```python
from build123d import *

# Parameters (mm, degrees)
SKETCH1_W                   = 31.75
SKETCH1_H                   = 8.89
SKETCH1_R                   = 2
BOSS_EXTRUDE1_DEPTH         = 2.54
SKETCH3_W                   = 2.54
SKETCH3_H                   = 8.89
BOSS_EXTRUDE2_DEPTH         = 27
SKETCH4_W                   = 17.08
SKETCH4_H                   = 2.54
CUT_EXTRUDE1_DEPTH          = 2.54
TAP_DRILL_FOR_M4X0_7_TAP1_D = 3.3


with BuildPart() as part:
    # Sketch1 → Boss-Extrude1 (new body)
    with BuildSketch(Plane.XY):
        with Locations((17.5, 25)):
            Rectangle(SKETCH1_W, SKETCH1_H)
        with Locations((17.5, 25)):
            Circle(SKETCH1_R, mode=Mode.SUBTRACT)
    extrude(amount=BOSS_EXTRUDE1_DEPTH)

    # Sketch3 → Boss-Extrude2 (add)
    with BuildSketch(Plane.XY.offset(2.54)):
        with Locations((10.23, 25)):
            Rectangle(SKETCH3_W, SKETCH3_H)
        with Locations((24.77, 25)):
            Rectangle(SKETCH3_W, SKETCH3_H)
    extrude(amount=BOSS_EXTRUDE2_DEPTH)

    # Sketch4 → Cut-Extrude1 (cut)
    with BuildSketch(Plane(origin=(0, 29.445, 0), x_dir=(1, 0, 0), z_dir=(0, 1, 0))):
        with Locations((17.5, -23.19)):
            Rectangle(SKETCH4_W, SKETCH4_H)
        with Locations((17.5, -14.3)):
            Rectangle(SKETCH4_W, SKETCH4_H)
    cut_extrude1 = extrude(amount=-CUT_EXTRUDE1_DEPTH, mode=Mode.SUBTRACT)

    # Mirror1: Cut-Extrude1 across plane
    add(cut_extrude1.mirror(Plane.ZX.offset(25)), mode=Mode.SUBTRACT)

    # Tap Drill for M4x0.7 Tap1 (through all)
    with Locations(Plane.XY.offset(2.54)):
        with Locations((4.8, 25), (30.2, 25)):
            Hole(TAP_DRILL_FOR_M4X0_7_TAP1_D / 2)


solid = part.part
```
Verification items for the finished model (mm, model axes). A direction names the side the tool comes from. Coordinates: 2 decimals unless noted, no trailing zeros. Loops run counter-clockwise (first coordinate to the right, second up) from the corner with the lowest first, then second, coordinate; pieces in that order, holes last. Notation, with made-up numbers: (80.5, -36.75) -> (96.5, -36.75) arc R17 cw to (96.5, -15.75) -> close; hole circle Ø7 at (29.5, 25). An arc over 180 degrees is marked (long way). Answer in a Markdown table with one row per item. Add a question column.
1. Section check D-D, the plane y = 21. Enter the section's corners in (x, z) (3 decimals).
2. Section check B-B, the plane x = 4.8. Enter the section's corners in (y, z) (3 decimals), then the cut area to 3 significant figures.
3. Material ranges on probe 1 along Z at (x, y) = (25.5, 22.5); probe 2 along Y at (x, z) = (30.2, 0.85) (3 decimals); probe 3 along Y at (x, z) = (17.5, 0.9) (3 decimals), recorded low to high. Write a range as [from, to].
4. Section check A-A, the plane z = 27.75. Enter the section's corners in (x, y) (3 decimals).
5. Access from +Z, -Z, +X, -X, +Y, -Y to the whole of each face (thin tool, end or side, straight path). Record for faces 1 (the face through (26.04, 25, 16)), 2 (the face through (25, 22, 21.92)), 3 (the face through (25, 26.905, 23)).
6. Depth check by flat-ended pin: P1, Ø2, axis at x = 25, y = 28.5, coming from the -Z side; P2, Ø5, axis at x = 29, y = 25, coming from the +Z side; P3, Ø2, axis at y = 24, z = 25, coming from the +X side; P4, Ø4, axis at y = 23.5, z = 15.5, coming from the -X side. Enter the tip coordinate at first touch or a pass-through.
7. Section check C-C, the plane y = 25. Enter the section's corners in (x, z) (3 decimals), then the cut area to 3 significant figures.
8. Draft check along Z on faces 4 (the face through (25, 28, 13.03)), 5 (the face through (25, 25, 29.54)), 6 (the face through (25, 20.555, 19)). Enter one of: +Z half, -Z half, draft (parallel to the pull), parting line (faces both ways), or undercut.
Derived:
| question | item | result |
|---|---|---|
| 1 | outline | (1.625, 0) -> (33.375, 0) -> (33.375, 2.54) -> (26.04, 2.54) -> (26.04, 13.03) -> (23.5, 13.03) -> (23.5, 2.54) -> (11.5, 2.54) -> (11.5, 13.03) -> (8.96, 13.03) -> (8.96, 2.54) -> (1.625, 2.54) -> close; (8.96, 15.57) -> (11.5, 15.57) -> (11.5, 21.92) -> (8.96, 21.92) -> close; (8.96, 24.46) -> (11.5, 24.46) -> (11.5, 29.54) -> (8.96, 29.54) -> close; (23.5, 15.57) -> (26.04, 15.57) -> (26.04, 21.92) -> (23.5, 21.92) -> close; (23.5, 24.46) -> (26.04, 24.46) -> (26.04, 29.54) -> (23.5, 29.54) -> close |
| 2 | outline | (20.555, 0) -> (23.35, 0) -> (23.35, 2.54) -> (20.555, 2.54) -> close; (26.65, 0) -> (29.445, 0) -> (29.445, 2.54) -> (26.65, 2.54) -> close |
| 2 | area | 14.2 mm² |
| 3 | probe 1 | z = [0, 13.03], [15.57, 21.92], [24.46, 29.54] |
| 3 | probe 2 | y = [20.555, 23.35], [26.65, 29.445] |
| 3 | probe 3 | y = [20.555, 23], [27, 29.445] |
| 4 | outline | (8.96, 20.555) -> (11.5, 20.555) -> (11.5, 29.445) -> (8.96, 29.445) -> close; (23.5, 20.555) -> (26.04, 20.555) -> (26.04, 29.445) -> (23.5, 29.445) -> close |
| 5 | face 1 | +Z, +X, +Y, -Y |
| 5 | face 2 | +X, -X, -Y |
| 5 | face 3 | +X, -X, +Y |
| 6 | P1 | stops at z = 0 |
| 6 | P2 | stops at z = 2.54 |
| 6 | P3 | stops at x = 26.04 |
| 6 | P4 | stops at x = 8.96 |
| 7 | outline | (1.625, 0) -> (3.15, 0) -> (3.15, 2.54) -> (1.625, 2.54) -> close; (6.45, 0) -> (15.5, 0) -> (15.5, 2.54) -> (11.5, 2.54) -> (11.5, 29.54) -> (8.96, 29.54) -> (8.96, 2.54) -> (6.45, 2.54) -> close; (19.5, 0) -> (28.55, 0) -> (28.55, 2.54) -> (26.04, 2.54) -> (26.04, 29.54) -> (23.5, 29.54) -> (23.5, 2.54) -> (19.5, 2.54) -> close; (31.85, 0) -> (33.375, 0) -> (33.375, 2.54) -> (31.85, 2.54) -> close |
| 7 | area | 191 mm² |
| 8 | face 4 | undercut |
| 8 | face 5 | +Z half |
| 8 | face 6 | draft |
